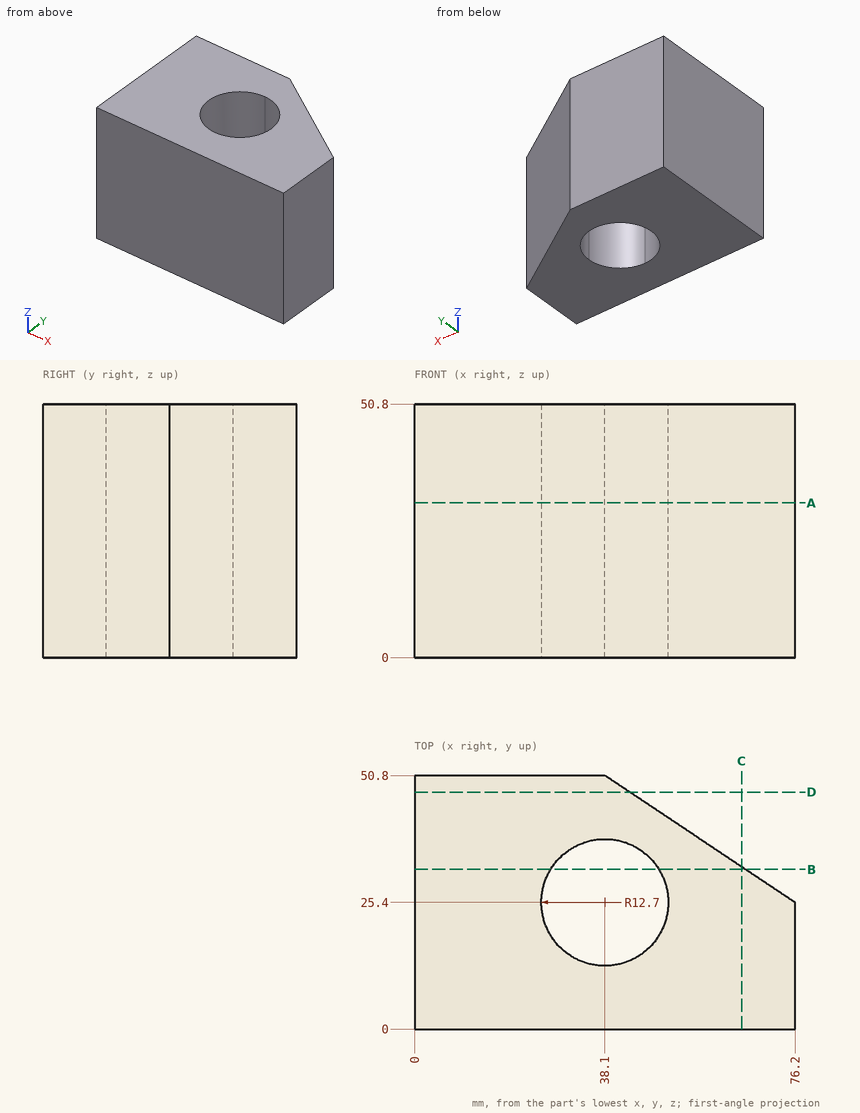
Input: dimensioned drawing with shaded views. Units: mm. Origin: part minimum x, y, z. Coordinates: 2 decimals unless noted, no trailing zeros. Loops run counter-clockwise (first coordinate to the right, second up) from the corner with the lowest first, then second, coordinate; pieces in that order, holes last. Notation, with made-up numbers: M 52,36.25 L 92,36.25 A17 ccw 92,45.25 Z; hole C 68.5,48 d4. An arc over 180 degrees is marked long. Use a Markdown table: item, result. Add a question column.
1) Pin query (flat end, axial travel): P1, Ø6, axis at y = 38, z = 36.5, coming from the +X side. Return the tip coordinate at first contact, or that it passes through.
2) Section C-C, the plane x = 65.5. Return the cut outline in (y, z).
3) Section A-A, the plane z = 31. Return the cut outline in (x, y).
4) Section D-D, the plane y = 47.5. Return the cut outline in (x, z), plus the area to 3 significant figures.
5) Section B-B, the plane y = 32. Return the cut outline in (x, z).
6) Line query: L1, parallel to X at y = 15, z = 39; L2, parallel to Y at x = 30, z = 43; L3, parallel to Y at x = 40, z = 36. Output: solid intervals per line, ascending. Write a range as from..to.
Answer below:
| question | item | result |
|---|---|---|
| 1 | P1 | x = 61.8 |
| 2 | outline | M 0,0 L 32.53,0 L 32.53,50.8 L 0,50.8 Z |
| 3 | outline | M 0,0 L 76.2,0 L 76.2,25.4 L 38.1,50.8 L 0,50.8 Z; hole C 38.1,25.4 d25.4 |
| 4 | outline | M 0,0 L 43.05,0 L 43.05,50.8 L 0,50.8 Z |
| 4 | area | 2,190 mm2 |
| 5 | outline | M 0,0 L 27.25,0 L 27.25,50.8 L 0,50.8 Z; M 48.95,0 L 66.3,0 L 66.3,50.8 L 48.95,50.8 Z |
| 6 | L1 | 0..30.81, 45.39..76.2 |
| 6 | L2 | 0..15.62, 35.18..50.8 |
| 6 | L3 | 0..12.84, 37.96..49.53 |
